The figure shows three views and two pictorial views of one solid part (mm, origin at its lowest corner). Answer the questions. Coordinates: 2 decimals unless noted, no trailing zeros. Write each loop counter-clockwise with the first axis right and the second up, starting at its lowest first coordinate (ties: lowest second). Pieces come first, ordered by that corner, then holes. Notation, with made-up numbers: M 35.5,65 L 68.5,65 A21 cw 68.5,77 Z; hole C -37.75,17 d5. An arc over 180 degrees is marked long. Use CSV: the item, a comma, the result in double quotes.
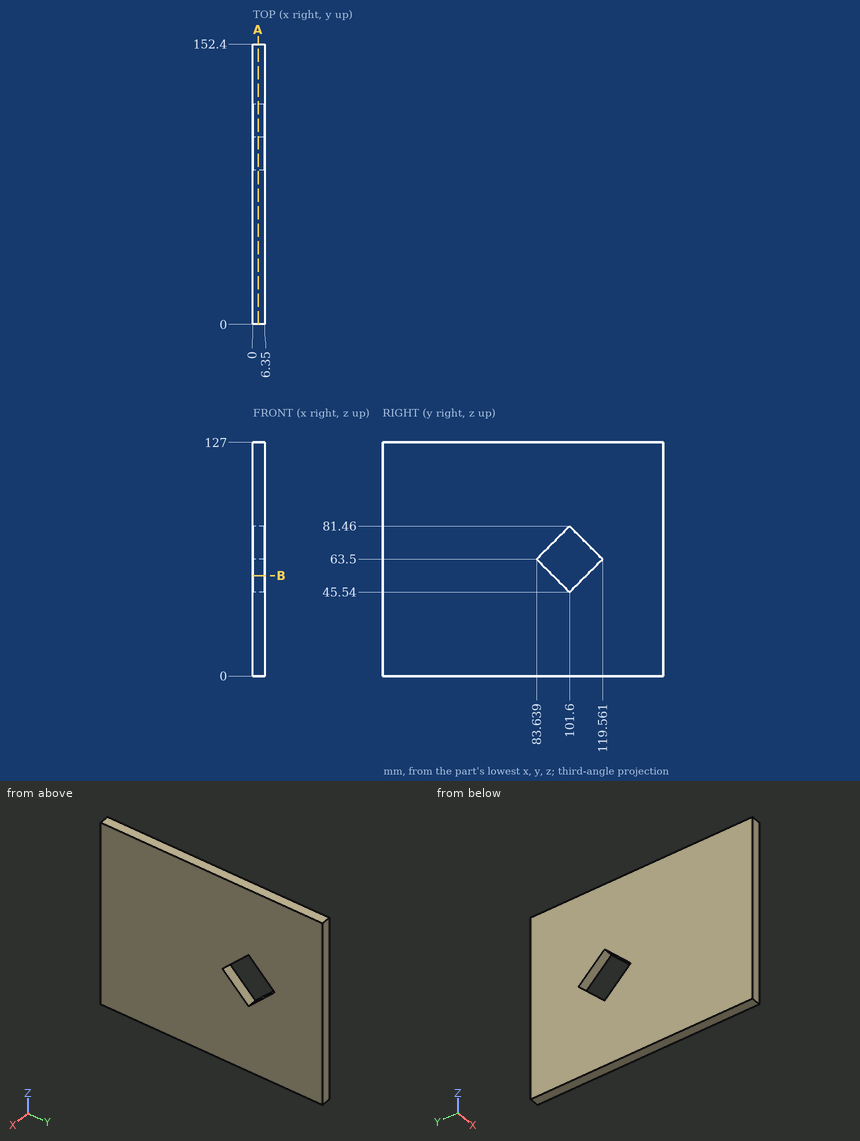
Item 1: The part is cut by section B-B (z = 54.5). Write down the section's boundary in (x, y).
Answer:
outline,"M 0,0 L 6.35,0 L 6.35,92.64 L 0,92.64 Z; M 0,110.56 L 6.35,110.56 L 6.35,152.4 L 0,152.4 Z"
Item 2: Consider probe 1 along Y at (x, z) = (4.75, 57); probe 2 along Y at (x, z) = (4.75, 69); probe 3 along Z at (x, y) = (1, 117.5). Determine where each line is inside the solid, lowest interval first.
Answer:
probe 1,"y = 0 to 90.14, 113.06 to 152.4"
probe 2,"y = 0 to 89.14, 114.06 to 152.4"
probe 3,"z = 0 to 61.44, 65.56 to 127"
Item 3: The part is cut by section A-A (x = 2.75). Write down the section's boundary in (y, z).
Answer:
outline,"M 0,0 L 152.4,0 L 152.4,127 L 0,127 Z; hole M 83.64,63.5 L 101.6,45.54 L 119.56,63.5 L 101.6,81.46 Z"
